```python
from build123d import *

# Parameters (mm, degrees)
SKETCH1_W           = 5
SKETCH1_H           = 5
BOSS_EXTRUDE1_DEPTH = 10
BOSS_EXTRUDE2_DEPTH = 5
BOSS_EXTRUDE3_DEPTH = 5
SKETCH4_R           = 5
BOSS_EXTRUDE4_DEPTH = 5
SKETCH5_R           = 4
BOSS_EXTRUDE5_DEPTH = 80
SKETCH6_W           = 4
SKETCH6_H           = 4
BOSS_EXTRUDE6_DEPTH = 4


with BuildPart() as part:
    # Sketch1 → Boss-Extrude1 (new body)
    with BuildSketch(Plane(origin=(0, 0, 0), x_dir=(1, 0, 0), z_dir=(0, 1, 0))):
        Rectangle(SKETCH1_W, SKETCH1_H)
    extrude(amount=BOSS_EXTRUDE1_DEPTH)

    # Sketch2 → Boss-Extrude2 (add)
    with BuildSketch(Plane.XZ):
        Polygon((0, 7.5), (-6.495190528, 3.75), (-6.495190528, -3.75), (0, -7.5), (6.495190528, -3.75), (6.495190528, 3.75), align=None)
    extrude(amount=BOSS_EXTRUDE2_DEPTH)

    # Sketch3 → Boss-Extrude3 (add)
    with BuildSketch(Plane(origin=(0, 10, 0), x_dir=(1, 0, 0), z_dir=(0, 1, 0))):
        Polygon((0, -7.5), (6.495190528, -3.75), (6.495190528, 3.75), (0, 7.5), (-6.495190528, 3.75), (-6.495190528, -3.75), align=None)
    extrude(amount=BOSS_EXTRUDE3_DEPTH)

    # Sketch4 → Boss-Extrude4 (add)
    with BuildSketch(Plane(origin=(0, 15, 0), x_dir=(1, 0, 0), z_dir=(0, 1, 0))):
        Circle(SKETCH4_R)
    extrude(amount=BOSS_EXTRUDE4_DEPTH)

    # Sketch5 → Boss-Extrude5 (add)
    with BuildSketch(Plane(origin=(0, 20, 0), x_dir=(1, 0, 0), z_dir=(0, 1, 0))):
        Circle(SKETCH5_R)
    extrude(amount=BOSS_EXTRUDE5_DEPTH)

    # Sketch6 → Boss-Extrude6 (add)
    with BuildSketch(Plane(origin=(0, 100, 0), x_dir=(1, 0, 0), z_dir=(0, 1, 0))):
        Rectangle(SKETCH6_W, SKETCH6_H)
    extrude(amount=BOSS_EXTRUDE6_DEPTH)


solid = part.part
```
Source: CAD feature listing. Evaluate the final solid. Frame: model axes, mm. A direction names the side the tool comes from. Round coordinates to 2 decimals unless told otherwise and drop trailing zeros. Loops run counter-clockwise (first coordinate to the right, second up) from the corner with the lowest first, then second, coordinate; pieces in that order, holes last. Notation, with made-up numbers: M 30,86.5 L 82,86.5 A16 ccw 82,93.5 Z; hole C -34,-5 d2. An arc over 180 degrees is marked long. Use a Markdown table: item, result. Add a question column.
1. Cut plane B-B, the plane y = 58.5. Output: boundary loops of the cut face in (x, z), and give its area (3 significant figures).
2. Contact query for flat-ended pins moving along their axis: pin 1 (6 mm diameter, centred on x = 2.5, y = 30, fed in from +Z); pin 2 (8 mm diameter, centred on y = 18, z = 5.5, fed in from +X); pin 3 (6 mm diameter, centred on y = 64, z = 1.5, fed in from -X); pin 4 (3 mm diameter, centred on x = 0, y = 102, fed in from +Z). Output: stop coordinate, or through.
3. Set-up query: faces 1 (the flat face through (2, 102, 0)), 2 (the flat face through (0, 5, -2.5)), 3 (the flat face through (0, 102, -2)). Return all of +Z, -Z, +X, -X, +Y, -Y with unobstructed straight access to the full face (end or side cutting, diameter ignored); none if empty.
4. Ray query, line 1 along Y through (x, z) = (2.5, -5.25); line 2 along Y through (x, z) = (-3.25, 0.5); line 3 along Y through (x, z) = (2.25, -2). Return the intervals inside material, ascending. Write a range as [from, to].
5. Pull-direction query (Y, two-part tool) for faces 4 (the flat face through (0, 104, 0)), 5 (the flat face through (-3.29, -2.46, -5.6)), 6 (the flat face through (0, 0, -3)); classes: +Y half, -Y half, draft (parallel to the pull), parting line (faces both ways), or undercut.
6. Cut plane A-A, the plane z = 0. Output: boundary loops of the cut face in (x, y), and give its area (3 significant figures).
Solution:
| question | item | result |
|---|---|---|
| 1 | outline | C 0,0 d8 |
| 1 | area | 50.3 mm2 |
| 2 | pin 1 | stops at z = 4 |
| 2 | pin 2 | stops at x = 6.5 |
| 2 | pin 3 | stops at x = -4 |
| 2 | pin 4 | stops at z = 2 |
| 3 | face 1 | +Z, -Z, +X, +Y |
| 3 | face 2 | -Z, +X, -X |
| 3 | face 3 | -Z, +X, -X, +Y |
| 4 | line 1 | y = [-5, 0], [10, 15] |
| 4 | line 2 | y = [-5, 0], [10, 100] |
| 4 | line 3 | y = [-5, 100] |
| 5 | face 4 | +Y half |
| 5 | face 5 | draft |
| 5 | face 6 | undercut |
| 6 | outline | M -6.5,-5 L 6.5,-5 L 6.5,0 L 2.5,0 L 2.5,10 L 6.5,10 L 6.5,15 L 5,15 L 5,20 L 4,20 L 4,100 L 2,100 L 2,104 L -2,104 L -2,100 L -4,100 L -4,20 L -5,20 L -5,15 L -6.5,15 L -6.5,10 L -2.5,10 L -2.5,0 L -6.5,0 Z |
| 6 | area | 886 mm2 |
